```python
from build123d import *

# Parameters (mm, degrees)
BOSS_EXTRUDE1_DEPTH     = 76.2
SKETCH2_R               = 3.175
CUT_EXTRUDE1_DEPTH      = 88.080358512
CUT_EXTRUDE1_DEPTH_BACK = 4.175
SKETCH4_R               = 3.175
CUT_EXTRUDE3_DEPTH      = 3.175


with BuildPart() as part:
    # Sketch1 → Boss-Extrude1 (new body)
    with BuildSketch(Plane(origin=(0, 0, 0), x_dir=(1, 0, 0), z_dir=(0, 1, 0))):
        with BuildLine():
            Line((-279.4, 0), (-279.4, 25.4))
            ThreePointArc((-279.4, 25.4), (-279.267281416, 26.691476594), (-278.874673451, 27.928968009))
            Line((-278.874673451, 27.928968009), (-192.844968037, 226.071031991))
            ThreePointArc((-192.844968037, 226.071031991), (-193.36014778, 232.083069992), (-198.669641488, 234.95))
            Line((-198.669641488, 234.95), (-269.875, 234.95))
            ThreePointArc((-269.875, 234.95), (-274.365128061, 233.090128061), (-276.225, 228.6))
            Line((-276.225, 228.6), (-276.225, 203.2))
            Line((-276.225, 203.2), (-279.4, 203.2))
            Line((-279.4, 203.2), (-279.4, 228.6))
            ThreePointArc((-279.4, 228.6), (-276.610192091, 235.335192091), (-269.875, 238.125))
            Line((-269.875, 238.125), (-198.669641488, 238.125))
            ThreePointArc((-198.669641488, 238.125), (-190.705400927, 233.824604988), (-189.932631312, 224.806547986))
            Line((-189.932631312, 224.806547986), (-275.962336725, 26.664484005))
            ThreePointArc((-275.962336725, 26.664484005), (-276.158640708, 26.045738297), (-276.225, 25.4))
            Line((-276.225, 25.4), (-276.225, 0))
            Line((-276.225, 0), (-279.4, 0))
        make_face()
    extrude(amount=BOSS_EXTRUDE1_DEPTH)

    # Sketch2 → Cut-Extrude1 (cut, two sides)
    with BuildSketch(Plane(origin=(-276.225, 0, 0), x_dir=(0, 0, -1), z_dir=(1, 0, 0))) as cut_extrude1_sk:
        with Locations((12.7, 63.5)):
            Circle(SKETCH2_R)
        with Locations((12.7, 12.7)):
            Circle(SKETCH2_R)
        with Locations((12.7, 38.1)):
            Circle(SKETCH2_R)
    extrude(amount=CUT_EXTRUDE1_DEPTH, mode=Mode.SUBTRACT)
    extrude(cut_extrude1_sk.sketch, amount=-CUT_EXTRUDE1_DEPTH_BACK, mode=Mode.SUBTRACT)

    # Sketch4 → Cut-Extrude3 (cut)
    with BuildSketch(Plane.ZY.offset(279.4)):
        with Locations((-215.9, 38.1)):
            Circle(SKETCH4_R)
        with Locations((-215.9, 63.5)):
            Circle(SKETCH4_R)
        with Locations((-215.9, 12.7)):
            Circle(SKETCH4_R)
    extrude(amount=-CUT_EXTRUDE3_DEPTH, mode=Mode.SUBTRACT)


solid = part.part
```
Source: CAD feature listing. Evaluate the final solid. Frame: model axes, mm. A direction names the side the tool comes from. Round coordinates to 2 decimals unless told otherwise and drop trailing zeros. Loops run counter-clockwise (first coordinate to the right, second up) from the corner with the lowest first, then second, coordinate; pieces in that order, holes last. Notation, with made-up numbers: (53, 21) - (105, 21) arc R26 cw to (105, 44) - close; hole circle Ø11 at (48, 78). An arc over 180 degrees is marked (long way). Use CSV: the item, a comma, the result in double quotes.
Q1. Mould query, pull axis Y, two halves, no side actions, for faces 1 (the cylindrical face through (-276.684, 37.567, -235.261)), 2 (the cylindrical face through (-277.79, 36.17, -10.18)), 3 (the cylindrical face through (-277.79, 65.646, -10.36)), 4 (the flat face through (-234, 76.2, -128)). Classes: pulls with the +Y half, pulls with the -Y half, needs draft (parallel to the pull), parting line crosses it, or undercut.
Reported:
face 1,"needs draft"
face 2,"undercut"
face 3,"undercut"
face 4,"pulls with the +Y half"
Q2. Section query A-A, the plane y = 12.7. Output: boundary loops of the cut face in (x, z) (3 decimals).
Reported:
outline,"(-279.4, -228.6) arc R9.525 ccw to (-269.875, -238.125) - (-198.67, -238.125) arc R9.525 ccw to (-189.933, -224.807) - (-275.962, -26.664) arc R3.175 cw to (-276.225, -25.4) - (-276.225, -15.875) - (-279.4, -15.875) - (-279.4, -25.4) arc R6.35 ccw to (-278.875, -27.929) - (-192.845, -226.071) arc R6.35 cw to (-198.67, -234.95) - (-269.875, -234.95) arc R6.35 cw to (-276.225, -228.6) - (-276.225, -219.075) - (-279.4, -219.075) - close; (-279.4, -212.725) - (-276.225, -212.725) - (-276.225, -203.2) - (-279.4, -203.2) - close; (-279.4, -9.525) - (-276.225, -9.525) - (-276.225, 0) - (-279.4, 0) - close"
Q3. Section query C-C, the plane z = -215.9. Output: boundary loops of the cut face in (x, y) (3 decimals), then the cut area to 3 significant figures.
Reported:
outline,"(-279.4, 0) - (-276.225, 0) - (-276.225, 9.525) - (-279.4, 9.525) - close; (-279.4, 15.875) - (-276.225, 15.875) - (-276.225, 34.925) - (-279.4, 34.925) - close; (-279.4, 41.275) - (-276.225, 41.275) - (-276.225, 60.325) - (-279.4, 60.325) - close; (-279.4, 66.675) - (-276.225, 66.675) - (-276.225, 76.2) - (-279.4, 76.2) - close; (-197.261, 0) - (-193.8, 0) - (-193.8, 76.2) - (-197.261, 76.2) - close"
area,"445 mm^2"
Q4. Pin query (flat end, axial travel): pin 1 Ø7.5 at (y, z) = (38.1, -12.7) entering from +X (3 decimals); pin 2 Ø5.5 at (y, z) = (12.7, -12.7) entering from -X; pin 3 Ø5 at (y, z) = (9, -74.5) entering from -X; pin 4 Ø12 at (x, z) = (-210.5, -169.5) entering from +Y. Return the tip coordinate at first contact, or that it passes through.
Reported:
pin 1,"x = -276.225"
pin 2,"through"
pin 3,"x = -259.74"
pin 4,"y = 76.2"
Q5. Section query B-B, the plane z = -12.7. Output: boundary loops of the cut face in (x, y) (3 decimals), then the cut area to 3 significant figures.
Reported:
outline,"(-279.4, 0) - (-276.225, 0) - (-276.225, 9.525) - (-279.4, 9.525) - close; (-279.4, 15.875) - (-276.225, 15.875) - (-276.225, 34.925) - (-279.4, 34.925) - close; (-279.4, 41.275) - (-276.225, 41.275) - (-276.225, 60.325) - (-279.4, 60.325) - close; (-279.4, 66.675) - (-276.225, 66.675) - (-276.225, 76.2) - (-279.4, 76.2) - close"
area,"181 mm^2"
Q6. Ray query, line 1 along Y through (x, z) = (-277.6, -215.9) (3 decimals); line 2 along Z through (x, y) = (-278, 38); line 3 along Z through (x, y) = (-277, 12). Return the intervals inside material, ascending.
Reported:
line 1,"0 to 9.525, 15.875 to 34.925, 41.275 to 60.325, 66.675 to 76.2"
line 2,"-233.57 to -219.07, -212.73 to -203.2, -29.94 to -15.87, -9.53 to 0"
line 3,"-234.92 to -219, -212.8 to -203.2, -32.25 to -15.8, -9.6 to 0"
Q7. Reachability of faces 5 (the cylindrical face through (-277.79, 10.77, -10.18)), 6 (the cylindrical face through (-274.315, 37.567, -233.139)), 7 (the flat face through (-276.225, 38, -7)), 8 (the cylindrical face through (-277.835, 66.177, -214.193)) from +Z, -Z, +X, -X, +Y, -Y: full face, straight path, thin tool, end or side. Return the list, or none.
Reported:
face 5,"+X, -X"
face 6,"+Y, -Y"
face 7,"+Z, +X, +Y, -Y"
face 8,"-X"
